For this review, use the dimensioned drawing (mm, ordinates from the lowest corner) and the shaded views. A direction names the side the tool comes from. Coordinates: 2 decimals unless noted, no trailing zeros. Write each loop counter-clockwise with the first axis right and the second up, starting at its lowest first coordinate (ties: lowest second). Pieces come first, ordered by that corner, then holes. Notation, with made-up numbers: (21.5, 42.5) - (74.5, 42.5) arc R26 ccw to (74.5, 60.5) - close; hole circle Ø10 at (26.5, 27). An arc over 180 degrees is marked (long way). One line per item, written item: value.
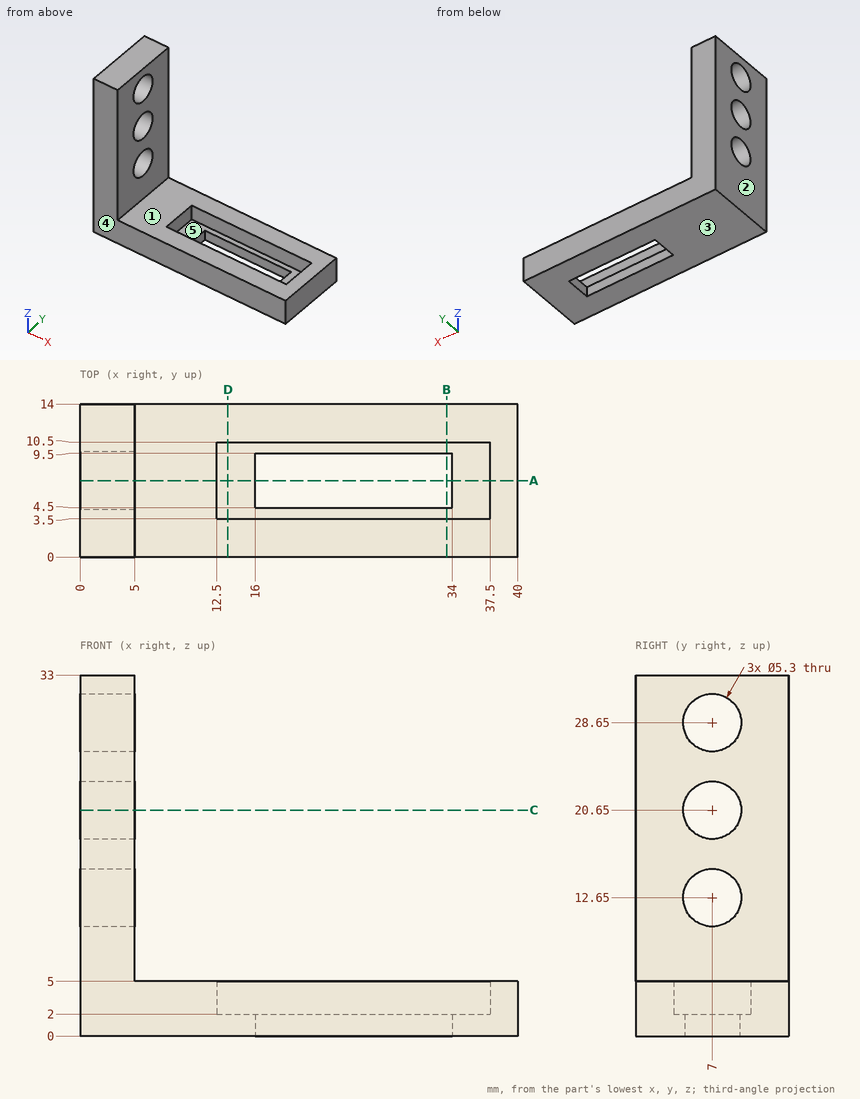
1. Mouldability with a two-part tool opening along Y and no side actions: class the marked faces 3, 4 and 5 as released by +Y, released by -Y, zero draft, split by the parting line, or undercut.
Answer block:
face 3: zero draft
face 4: released by -Y
face 5: undercut
2. Consider section C-C, the plane z = 20.65. Write out the cut boundary in (x, y), then the cut area to 3 significant figures.
Answer block:
outline: (0, 0) - (5, 0) - (5, 4.35) - (0, 4.35) - close; (0, 9.65) - (5, 9.65) - (5, 14) - (0, 14) - close
area: 43.5 mm^2
3. Wall thickness on line 1 along Y through (x, z) = (2, 20.65); line 2 along X through (y, z) = (7, 3.5); line 3 along X through (y, z) = (7, 6.5): over which ranges is each line inside the solid? List them lowest first.
Answer block:
line 1: y = 0 to 4.35, 9.65 to 14
line 2: x = 0 to 12.5, 37.5 to 40
line 3: x = 0 to 5
4. For the marked faces 1 and 2, list the 3-axis set-ups (+Z, -Z, +X, -X, +Y, -Y) from which the entire face can be reached by the end or side of a thin tool; tool diameter is ignored.
Answer block:
face 1: +Z, +X, +Y, -Y
face 2: +Z, -Z, -X, +Y, -Y
5. Consider section A-A, the plane y = 7. Write out the cut boundary in (x, z).
Answer block:
outline: (0, 0) - (16, 0) - (16, 2) - (12.5, 2) - (12.5, 5) - (5, 5) - (5, 10) - (0, 10) - close; (0, 15.3) - (5, 15.3) - (5, 18) - (0, 18) - close; (0, 23.3) - (5, 23.3) - (5, 26) - (0, 26) - close; (0, 31.3) - (5, 31.3) - (5, 33) - (0, 33) - close; (34, 0) - (40, 0) - (40, 5) - (37.5, 5) - (37.5, 2) - (34, 2) - close
6. Insertion check: pin 1 Ø2 at (y, z) = (8, 1.5) entering from -X; pin 2 Ø7 at (x, y) = (23, 5) entering from +Z; pin 3 Ø3 at (y, z) = (7, 28.65) entering from +X; pin 4 Ø7 at (y, z) = (10, 24.5) entering from +X. Each pin has a flat end and moves straight along its axis. Give the tip position at first contact, or say it passes through.
Answer block:
pin 1: stops at x = 0
pin 2: stops at z = 5
pin 3: passes through
pin 4: stops at x = 5
7. Consider section B-B, the plane x = 33.5. Write out the cut boundary in (y, z).
Answer block:
outline: (0, 0) - (4.5, 0) - (4.5, 2) - (3.5, 2) - (3.5, 5) - (0, 5) - close; (9.5, 0) - (14, 0) - (14, 5) - (10.5, 5) - (10.5, 2) - (9.5, 2) - close
8. Consider section D-D, the plane x = 13.5. Write out the cut boundary in (y, z).
Answer block:
outline: (0, 0) - (14, 0) - (14, 5) - (10.5, 5) - (10.5, 2) - (3.5, 2) - (3.5, 5) - (0, 5) - close
